Geometry check sheet. Reference: the model listing, model coordinates, mm. Round coordinates to 2 decimals unless told otherwise and drop trailing zeros. Order: outer loops, then holes, each group sorted by start corner. A loop starts at its lowest first (then second) coordinate and runs counter-clockwise, first axis right, second up. Notation, with made-up numbers: (83.5, 20) -> (122.5, 20) arc R15 ccw to (122.5, 27) -> close; hole circle Ø3 at (-24, 62). An arc over 180 degrees is marked (long way). Use a Markdown table: item, result. Add a question column.
Item 1: Sectioned sample at D-D, the plane z = -70.5. Record the cut outline in (x, y) (3 decimals).
Item 2: Sectioned sample at A-A, the plane y = 27.8. Record the cut outline in (x, z) (3 decimals).
Item 3: Sectioned sample at B-B, the plane z = -11. Record the cut outline in (x, y) (3 decimals), and give its area (3 significant figures).
Item 4: Material ranges on probe 1 along Z at (x, y) = (0.3, 27.5); probe 2 along Y at (x, z) = (0.5, -72.5); probe 3 along Y at (x, z) = (1.2, -13.5), recorded low to high. Write a range as [from, to].
Item 5: Sectioned sample at C-C, the plane x = 1.65. Record the cut outline in (y, z) (3 decimals), and give its area (3 significant figures).
Item 6: Gauge pin test, flat ends, axial feed: pin 1 Ø1 at (x, y) = (2.5, 58.5) entering from -Z; pin 2 Ø1 at (x, z) = (1, -21.5) entering from +Y. Record the tip position at first contact, or that the pin passes through.
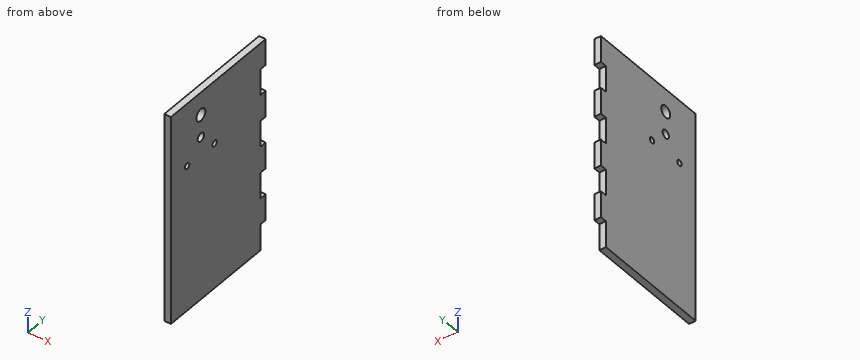
from build123d import *

# Parameters (mm, degrees)
BOSS_EXTRUDE1_DEPTH = 3.175
CUT_EXTRUDE1_REACH  = 5.175
SKETCH2_R           = 1.4
SKETCH2_R_2         = 2
SKETCH2_R_3         = 2.876999961


with BuildPart() as part:
    # Sketch1 → Boss-Extrude1 (new body)
    with BuildSketch(Plane(origin=(0, 0, 0), x_dir=(0, 0, -1), z_dir=(1, 0, 0))):
        Polygon((0, 0), (0, 60.325), (12.7, 60.325), (12.7, 57.15), (25.4, 57.15), (25.4, 60.325), (38.1, 60.325), (38.1, 57.15), (50.8, 57.15), (50.8, 60.325), (63.5, 60.325), (63.5, 57.15), (76.2, 57.15), (76.2, 60.325), (88.9, 60.325), (88.9, 57.15), (101.6, 57.15), (101.6, 0), align=None)
    extrude(amount=BOSS_EXTRUDE1_DEPTH)

    # Sketch2 → Cut-Extrude1 (cut, up to next)
    with BuildSketch(Plane(origin=(3.175, 0, 0), x_dir=(0, 0, -1), z_dir=(1, 0, 0)), mode=Mode.PRIVATE) as cut_extrude1_sk1:
        with Locations((30.59102, 10.3)):
            Circle(SKETCH2_R)
    cut_extrude1_tool1 = extrude(cut_extrude1_sk1.sketch, amount=-CUT_EXTRUDE1_REACH, mode=Mode.PRIVATE) & part.part
    add(cut_extrude1_tool1.solids().sort_by_distance((3.175, 10.3, -30.59102))[0], mode=Mode.SUBTRACT)
    # Sketch2 → Cut-Extrude1 (cut, up to next)
    with BuildSketch(Plane(origin=(3.175, 0, 0), x_dir=(0, 0, -1), z_dir=(1, 0, 0)), mode=Mode.PRIVATE) as cut_extrude1_sk2:
        with Locations((30.59102, 27.8)):
            Circle(SKETCH2_R)
    cut_extrude1_tool2 = extrude(cut_extrude1_sk2.sketch, amount=-CUT_EXTRUDE1_REACH, mode=Mode.PRIVATE) & part.part
    add(cut_extrude1_tool2.solids().sort_by_distance((3.175, 27.8, -30.59102))[0], mode=Mode.SUBTRACT)
    # Sketch2 → Cut-Extrude1 (cut, up to next)
    with BuildSketch(Plane(origin=(3.175, 0, 0), x_dir=(0, 0, -1), z_dir=(1, 0, 0)), mode=Mode.PRIVATE) as cut_extrude1_sk3:
        with Locations((22.0000034, 19.05)):
            Circle(SKETCH2_R_2)
    cut_extrude1_tool3 = extrude(cut_extrude1_sk3.sketch, amount=-CUT_EXTRUDE1_REACH, mode=Mode.PRIVATE) & part.part
    add(cut_extrude1_tool3.solids().sort_by_distance((3.175, 19.05, -22.000003))[0], mode=Mode.SUBTRACT)
    # Sketch2 → Cut-Extrude1 (cut, up to next)
    with BuildSketch(Plane(origin=(3.175, 0, 0), x_dir=(0, 0, -1), z_dir=(1, 0, 0)), mode=Mode.PRIVATE) as cut_extrude1_sk4:
        with Locations((11, 19.05)):
            Circle(SKETCH2_R_3)
    cut_extrude1_tool4 = extrude(cut_extrude1_sk4.sketch, amount=-CUT_EXTRUDE1_REACH, mode=Mode.PRIVATE) & part.part
    add(cut_extrude1_tool4.solids().sort_by_distance((3.175, 19.05, -11))[0], mode=Mode.SUBTRACT)


solid = part.part
Found:
| question | item | result |
|---|---|---|
| 1 | outline | (0, 0) -> (3.175, 0) -> (3.175, 57.15) -> (0, 57.15) -> close |
| 2 | outline | (0, -101.6) -> (3.175, -101.6) -> (3.175, -31.991) -> (0, -31.991) -> close; (0, -29.191) -> (3.175, -29.191) -> (3.175, 0) -> (0, 0) -> close |
| 3 | outline | (0, 0) -> (3.175, 0) -> (3.175, 16.173) -> (0, 16.173) -> close; (0, 21.927) -> (3.175, 21.927) -> (3.175, 60.325) -> (0, 60.325) -> close |
| 3 | area | 173 mm2 |
| 4 | probe 1 | z = [-101.6, -31.96], [-29.22, 0] |
| 4 | probe 2 | y = [0, 57.15] |
| 4 | probe 3 | y = [0, 17.63], [20.47, 57.15] |
| 5 | outline | (0, -101.6) -> (57.15, -101.6) -> (57.15, -88.9) -> (60.325, -88.9) -> (60.325, -76.2) -> (57.15, -76.2) -> (57.15, -63.5) -> (60.325, -63.5) -> (60.325, -50.8) -> (57.15, -50.8) -> (57.15, -38.1) -> (60.325, -38.1) -> (60.325, -25.4) -> (57.15, -25.4) -> (57.15, -12.7) -> (60.325, -12.7) -> (60.325, 0) -> (0, 0) -> close; hole circle Ø2.8 at (10.3, -30.591); hole circle Ø5.754 at (19.05, -11); hole circle Ø4 at (19.05, -22); hole circle Ø2.8 at (27.8, -30.591) |
| 5 | area | 5,920 mm2 |
| 6 | pin 1 | stops at z = -88.9 |
| 6 | pin 2 | stops at y = 57.15 |
